Build history of the part. All positions in model axes, mm. A direction names the side the tool comes from. Give positions to 0.01 mm unless a question says otherwise; leave off trailing zeros. Order: outer loops, then holes, each group sorted by start corner. A loop starts at its lowest first (then second) coordinate and runs counter-clockwise, first axis right, second up. Notation, with made-up numbers: (-40, -37.5) - (-13, -37.5) arc R19 cw to (-13, -22.5) - close; hole circle Ø3 at (-21, 43). An arc over 180 degrees is marked (long way). Write each question's results on one line, items separated by ' | '. Start each with the question number.
from build123d import *

# Parameters (mm, degrees)
SKETCH1_R           = 2.6
BOSS_EXTRUDE1_DEPTH = 2.5
FILLET1_R           = 0.3
SKETCH2_R           = 1.5
BOSS_EXTRUDE2_DEPTH = 5.5
FILLET2_R           = 0.2


with BuildPart() as part:
    # Sketch1 → Boss-Extrude1 (new body)
    with BuildSketch(Plane.XY):
        Circle(SKETCH1_R)
    extrude(amount=BOSS_EXTRUDE1_DEPTH)

    # Fillet1
    fillet1_edges = [part.edges().sort_by_distance(p)[0] for p in [
        (-2.6, 0, 0),
    ]]
    fillet(fillet1_edges, radius=FILLET1_R)

    # Sketch2 → Boss-Extrude2 (add)
    with BuildSketch(Plane.XY.offset(2.5)):
        Circle(SKETCH2_R)
    extrude(amount=BOSS_EXTRUDE2_DEPTH)

    # Fillet2
    fillet2_edges = [part.edges().sort_by_distance(p)[0] for p in [
        (-1.5, 0, 8),
    ]]
    fillet(fillet2_edges, radius=FILLET2_R)


solid = part.part
Item 1: Flat gauge pins, fed straight in: pin 1 Ø1.5 at (x, y) = (0, -1) entering from -Z; pin 2 Ø1 at (y, z) = (-1.5, 2.5) entering from -X; pin 3 Ø3 at (x, z) = (2, 4.5) entering from -Y. Where does each tip first touch, or does it go through?
Item 2: Cut at A-A, the plane y = 0. List the corners of the cut face in (x, z).
Item 3: Cut at C-C, the plane z = 7.5. List the corners of the cut face in (x, y).
Item 4: Probe line 1 along Z through (x, y) = (-1.7, 1.05); line 2 along X through (y, z) = (1, 4.5); line 3 along Y through (x, z) = (1.5, 0.5). List the from-to ranges inside material, lowest first. Write a range as from..to.
Item 5: Cut at D-D, the plane z = 2.25. List the corners of the cut face in (x, y), then the cut area to 3 significant figures.
Item 6: Which spindle directions (+Z, -Z, +X, -X, +Y, -Y) get a long thin tool onto all of the face, cutting with end or side? Do faces 1 (the cylindrical face through (-0.338, 2.578, 1.385)), 2 (the cylindrical face through (-1.5, 0.07, 5.11)). Say none if no direction does.
Values found:
1) pin 1: stops at z = 0 | pin 2: stops at x = -2.4 | pin 3: stops at y = -1.41
2) outline: (-2.6, 0.3) arc R0.3 ccw to (-2.3, 0) - (2.3, 0) arc R0.3 ccw to (2.6, 0.3) - (2.6, 2.5) - (1.5, 2.5) - (1.5, 7.8) arc R0.2 ccw to (1.3, 8) - (-1.3, 8) arc R0.2 ccw to (-1.5, 7.8) - (-1.5, 2.5) - (-2.6, 2.5) - close
3) outline: circle Ø3 at (0, 0)
4) line 1: z = 0..2.5 | line 2: x = -1.12..1.12 | line 3: y = -2.12..2.12
5) outline: circle Ø5.2 at (0, 0) | area: 21.2 mm2
6) face 1: +Z, -Z | face 2: +Z
